Input: dimensioned drawing with shaded views. Units: mm. Origin: part minimum x, y, z. A direction names the side the tool comes from. Coordinates: 2 decimals unless noted, no trailing zeros. Loops run counter-clockwise (first coordinate to the right, second up) from the corner with the lowest first, then second, coordinate; pieces in that order, holes last.
Item 1: Pull-direction query (Y, two-part tool) for the marked faces 1, 2 and 3; classes: +Y half, -Y half, draft (parallel to the pull), parting line (faces both ways), or undercut.
Item 2: Reachability of the marked faces 4 and 5 from +Z, -Z, +X, -X, +Y, -Y: full face, straight path, thin tool, end or side. Return the list, or none.
Item 3: Section query A-A, the plane x = 28. Return the cut outline in (y, z).
Item 4: Section query B-B, the plane y = 17.5. Return the cut outline in (x, z), then the cut area to 3 significant figures.
Item 5: Section query D-D, the plane z = 2.5. Return the cut outline in (x, y), then the cut area to 3 significant figures.
Item 6: Line query: probe 1 along Y at (x, z) = (19, 0.5); probe 2 along Z at (x, y) = (3, 29); probe 3 along Y at (x, z) = (31, 9). Output: solid intervals per line, ascending.
Item 7: Section query C-C, the plane y = 31.5. Return the cut outline in (x, z), then the cut area to 3 significant figures.
Item 8: Pin query (flat end, axial travel): pin 1 Ø13.5 at (x, y) = (19, 19) entering from +Z; pin 2 Ø4 at (x, z) = (4.5, 3.5) entering from -Y; pin 3 Ø4 at (x, z) = (29, 2.5) entering from -Y; pin 4 Ø3 at (x, z) = (18, 5.5) entering from -Y. Return the tip coordinate at first contact, or that it passes through.
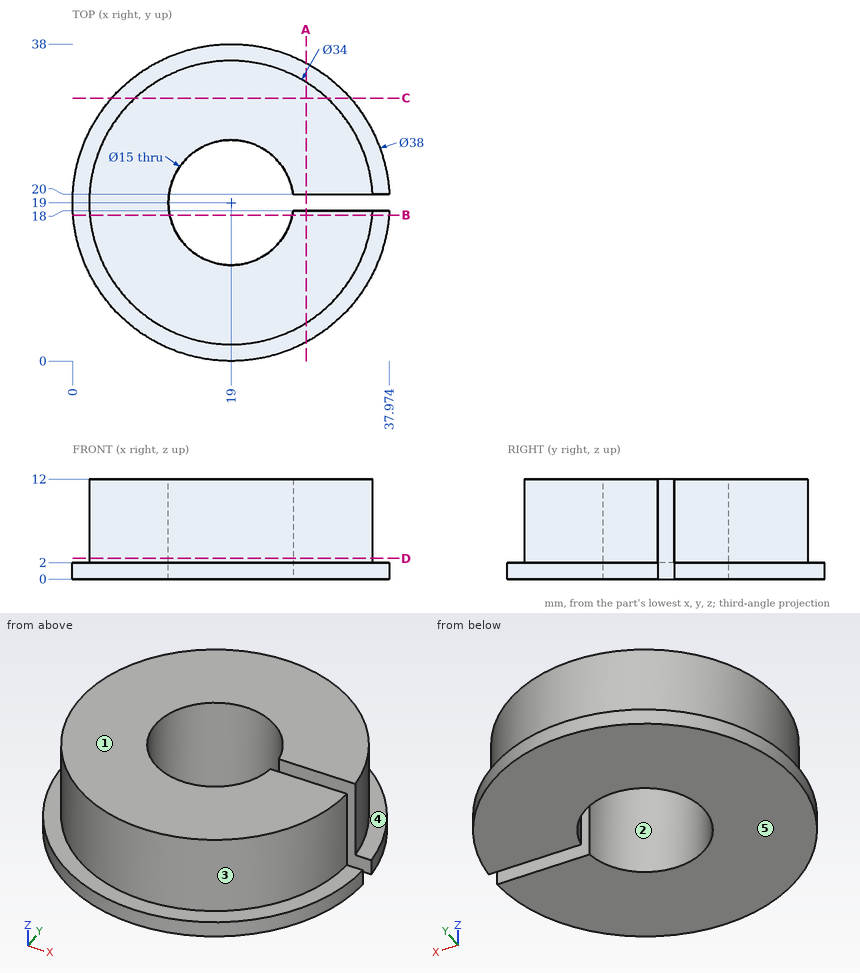
Verdict:
1. face 1: draft
1. face 2: undercut
1. face 3: parting line
2. face 4: +Z
2. face 5: -Z, +X, -X, +Y, -Y
3. outline: (2.27, 0) - (18, 0) - (18, 12) - (4.58, 12) - (4.58, 2) - (2.27, 2) - close; (20, 0) - (35.73, 0) - (35.73, 2) - (33.42, 2) - (33.42, 12) - (20, 12) - close
4. outline: (0.06, 0) - (11.65, 0) - (11.65, 12) - (2.07, 12) - (2.07, 2) - (0.06, 2) - close; (26.35, 0) - (37.94, 0) - (37.94, 2) - (35.93, 2) - (35.93, 12) - (26.35, 12) - close
4. area: 238 mm2
5. outline: (26.43, 18) arc R7.5 cw (long way) to (26.43, 20) - (35.97, 20) arc R17 ccw (long way) to (35.97, 18) - close
5. area: 712 mm2
6. probe 1: y = 0 to 11.5, 26.5 to 38
6. probe 2: z = 0 to 2
6. probe 3: y = 6.96 to 18, 20 to 31.04
7. outline: (4.69, 0) - (33.31, 0) - (33.31, 2) - (30.52, 2) - (30.52, 12) - (7.48, 12) - (7.48, 2) - (4.69, 2) - close
7. area: 288 mm2
8. pin 1: passes through
8. pin 2: stops at y = 5.31
8. pin 3: stops at y = 1.8
8. pin 4: stops at y = 2
